from build123d import *

# Parameters (mm, degrees)
F_1_4_20_TAPPED_HOLE1_D     = 5.1054
F_1_4_20_TAPPED_HOLE1_DEPTH = 8.118183098
F_1_4_20_TAPPED_HOLE1_TIP   = 1.533816902


with BuildPart() as part:
    # Sketch1 → Revolve1 (revolve)
    with BuildSketch(Plane.XY, mode=Mode.PRIVATE) as revolve1_sk:
        Polygon((0, 0), (22.225, 0), (22.225, -3.175), (47.498, -3.175), (47.498, -5.715), (44.577, -5.715), (44.577, -10.6934), (47.498, -10.6934), (47.498, -28.7782), (47.498, -33.7566), (47.498, -43.2816), (44.577, -43.2816), (44.577, -48.26), (47.498, -48.26), (47.498, -50.8), (41.148, -50.8), (41.148, -12.7), (0, -12.7), align=None)
    revolve(revolve1_sk.sketch.rotate(Axis((0, 38.901080227, 0), (0, -1, 0)), 180), axis=Axis((0, 38.901080227, 0), (0, -1, 0)))

    # 1/4-20 Tapped Hole1
    with Locations(Plane(origin=(0, 0, 0), x_dir=(1, 0, 0), z_dir=(0, 1, 0))):
        with Locations((0, 0)):
            Hole(F_1_4_20_TAPPED_HOLE1_D / 2, depth=F_1_4_20_TAPPED_HOLE1_DEPTH)
            with Locations((0, 0, -(F_1_4_20_TAPPED_HOLE1_DEPTH + F_1_4_20_TAPPED_HOLE1_TIP / 2))):  # 118° drill point
                Cone(0, F_1_4_20_TAPPED_HOLE1_D / 2, F_1_4_20_TAPPED_HOLE1_TIP, mode=Mode.SUBTRACT)


solid = part.part
For this review, take the finished solid that the model builds, in its own axes (mm). A direction names the side the tool comes from. Round coordinates to 2 decimals unless told otherwise and drop trailing zeros. Write each loop counter-clockwise with the first axis right and the second up, starting at its lowest first coordinate (ties: lowest second). Pieces come first, ordered by that corner, then holes. Notation, with made-up numbers: M 6,-27.5 L 19,-27.5 A11 ccw 19,-19.5 Z; hole C 7,44 d10. An arc over 180 degrees is marked long. Write item = value, one per line. Start each with the question number.
(1) The part is to be moulded in two halves that separate along Y. For faces 4 (the face through (32.855, -45.806, -30.127)), 5 (the face through (14, -50.8, -39)), 6 (the face through (-2.435, -4.116, -0.767)), say which applies: +Y half, -Y half, draft (parallel to the pull), parting line (faces both ways), or undercut.
(2) We need section A-A (y = -39.5). Give the boundary of the cut face in (x, z).
(3) For faces 1 (the face through (20.4, -3.175, 9.9)), 2 (the face through (32.855, -8.239, -30.127)), 3 (the face through (5.357, -31.483, -40.798)), list the 3-axis set-ups (+Z, -Z, +X, -X, +Y, -Y) from which the entire face can be reached by the end or side of a thin tool; tool diameter is ignored.
(4) Clearance check with flat-ended pins moving along their axes: pin 1 Ø10 at (x, z) = (4, 12) entering from -Y; pin 2 Ø3 at (x, y) = (22, -34) entering from -Z; pin 3 Ø3 at (x, z) = (-26.5, -26.5) entering from +Y (3 decimals). State where each tip first meets the part, or that it passes through.
(5) We need section B-B (x = 25). Give the boundary of the cut face in (y, z) (3 decimals).
(6) We need section C-C (z = 14). Give the boundary of the cut face in (x, y) (1 decimal), then the cut area to 3 significant figures.
(7) For line 1 along X through (y, z) = (-43.5, -21); line 2 along X through (y, z) = (-33, 1); line 3 along Y through (x, z) = (13, 28) (3 decimals), list the stretches that pass through material, from the lowest coordinate up.
(8) We need section D-D (x = 7). Give the boundary of the cut face in (y, z) (3 decimals), then the cut area to 3 significant figures.
Results found:
q1.face_4 = undercut
q1.face_5 = -Y half
q1.face_6 = draft
q2.outline = C 0,0 d95; hole C 0,0 d82.3
q3.face_1 = +Y
q3.face_2 = none
q3.face_3 = -Y
q4.pin_1 = -12.7
q4.pin_2 = -42.85
q4.pin_3 = -3.175
q5.outline = M -50.8,-40.386 L -48.26,-40.386 L -48.26,-36.907 L -43.282,-36.907 L -43.282,-40.386 L -10.693,-40.386 L -10.693,-36.907 L -5.715,-36.907 L -5.715,-40.386 L -3.175,-40.386 L -3.175,40.386 L -5.715,40.386 L -5.715,36.907 L -10.693,36.907 L -10.693,40.386 L -43.282,40.386 L -43.282,36.907 L -48.26,36.907 L -48.26,40.386 L -50.8,40.386 L -50.8,32.683 L -12.7,32.683 L -12.7,-32.683 L -50.8,-32.683 Z
q6.outline = M -45.4,-50.8 L -38.7,-50.8 L -38.7,-12.7 L 38.7,-12.7 L 38.7,-50.8 L 45.4,-50.8 L 45.4,-48.3 L 42.3,-48.3 L 42.3,-43.3 L 45.4,-43.3 L 45.4,-10.7 L 42.3,-10.7 L 42.3,-5.7 L 45.4,-5.7 L 45.4,-3.2 L 17.3,-3.2 L 17.3,0 L -17.3,0 L -17.3,-3.2 L -45.4,-3.2 L -45.4,-5.7 L -42.3,-5.7 L -42.3,-10.7 L -45.4,-10.7 L -45.4,-43.3 L -42.3,-43.3 L -42.3,-48.3 L -45.4,-48.3 Z
q6.area = 1,420 mm²
q7.line_1 = -39.32 to -35.39, 35.39 to 39.32
q7.line_2 = -47.49 to -41.14, 41.14 to 47.49
q7.line_3 = -12.7 to -3.175
q8.outline = M -50.8,-46.979 L -48.26,-46.979 L -48.26,-44.024 L -43.282,-44.024 L -43.282,-46.979 L -10.693,-46.979 L -10.693,-44.024 L -5.715,-44.024 L -5.715,-46.979 L -3.175,-46.979 L -3.175,-21.094 L 0,-21.094 L 0,21.094 L -3.175,21.094 L -3.175,46.979 L -5.715,46.979 L -5.715,44.024 L -10.693,44.024 L -10.693,46.979 L -43.282,46.979 L -43.282,44.024 L -48.26,44.024 L -48.26,46.979 L -50.8,46.979 L -50.8,40.548 L -12.7,40.548 L -12.7,-40.548 L -50.8,-40.548 Z
q8.area = 1,460 mm²
